```python
from build123d import *

# Parameters (mm, degrees)
ESQUISSE1_W             = 40
ESQUISSE1_H             = 40
BOSS_EXTRU_1_DEPTH      = 25
CHANFREIN1_SIZE         = 20
CHANFREIN1_SIZE2        = 11.547005384
ESQUISSE2_W             = 15
ESQUISSE2_H             = 15
ENL_V_MAT_EXTRU_1_DEPTH = 2


with BuildPart() as part:
    # Esquisse1 → Boss.-Extru.1 (new body)
    with BuildSketch(Plane(origin=(0, 0, 0), x_dir=(1, 0, 0), z_dir=(0, 1, 0))):
        Rectangle(ESQUISSE1_W, ESQUISSE1_H)
    extrude(amount=BOSS_EXTRU_1_DEPTH)

    # Chanfrein1
    chanfrein1_edges = [part.edges().sort_by_distance(p)[0] for p in [
        (20, 25, 0),
    ]]
    chanfrein1_side = [part.faces().sort_by_distance(p)[0] for p in [
        (20, 12.5, 0),
    ]]
    chamfer(chanfrein1_edges, length=CHANFREIN1_SIZE, length2=CHANFREIN1_SIZE2, reference=chanfrein1_side[0])

    # Esquisse2 → Enlèv. mat.-Extru.1 (cut)
    with BuildSketch(Plane(origin=(17.165063509, 9.910254038, 0), x_dir=(0, 0, -1), z_dir=(0.8660254037844397, 0.4999999999999983, 0))):
        with Locations((0, 5.877132403)):
            Rectangle(ESQUISSE2_W, ESQUISSE2_H)
    extrude(amount=-ENL_V_MAT_EXTRU_1_DEPTH, mode=Mode.SUBTRACT)


solid = part.part
```
Part model, mm, in its own coordinate system. A direction names the side the tool comes from. Round coordinates to 2 decimals unless told otherwise and drop trailing zeros. Loops run counter-clockwise (first coordinate to the right, second up) from the corner with the lowest first, then second, coordinate; pieces in that order, holes last. Notation, with made-up numbers: (18.25, 14.5) -> (66.25, 14.5) arc R6 cw to (66.25, 19.5) -> close; hole circle Ø2 at (3, 68). An arc over 180 degrees is marked (long way). Use CSV: the item, a comma, the result in double quotes. Start each with the question number.
1) Cut at B-B, the plane y = 17.5. Write the cut outline in (x, z), plus the area to 3 significant figures.
2) Cut at D-D, the plane z = -10. Write the cut outline in (x, y).
3) Pull direction Z, two halves, no side cores. Call faces 1 (the flat face through (13, 14, 7.5)), 2 (the flat face through (-20, 12, 0)), 3 (the flat face through (0, 12, 20)): +Z half, -Z half, draft (parallel to the pull), parting line (faces both ways), or undercut.
4) Drop a flat-ended pin along its axis: P1, Ø1, axis at y = 9, z = 14, coming from the +X side. Give the stop position or say it passes through.
5) Wall check: L1, parallel to Z at x = 13, y = 14; L2, parallel to X at y = 14.25, z = 7; L3, parallel to Y at x = 18, z = 14. Give the ranges that are in metal, low to high. Write a range as [from, to].
6) Cut at C-C, the plane x = 17. Write the cut outline in (y, z).
7) Cut at A-A, the plane z = -4.5. Write the cut outline in (x, y).
8) Which spindle directions (+Z, -Z, +X, -X, +Y, -Y) get a long thin tool onto all of the face, cutting with end or side? Do faces 4 (the flat face through (0, 12, -20)), 5 (the flat face through (17.1, 8, 0.1)), 6 (the flat face through (9.62, 21, 0.1)). Say none if no direction does.
Determined:
1,outline,"(-20, -20) -> (12.78, -20) -> (12.78, -7.5) -> (10.47, -7.5) -> (10.47, 7.5) -> (12.78, 7.5) -> (12.78, 20) -> (-20, 20) -> close"
1,area,"1,280 mm2"
2,outline,"(-20, 0) -> (20, 0) -> (20, 5) -> (8.45, 25) -> (-20, 25) -> close"
3,face 1,"undercut"
3,face 2,"draft"
3,face 3,"+Z half"
4,P1,"stops at x = 17.98"
5,L1,"z = [-20, -7.5], [7.5, 20]"
5,L2,"x = [-20, 12.35]"
5,L3,"y = [0, 8.46]"
6,outline,"(0, -20) -> (10.2, -20) -> (10.2, -7.5) -> (7.94, -7.5) -> (7.94, 7.5) -> (10.2, 7.5) -> (10.2, 20) -> (0, 20) -> close"
7,outline,"(-20, 0) -> (20, 0) -> (20, 5) -> (17.98, 8.5) -> (16.24, 7.5) -> (8.74, 20.5) -> (10.48, 21.5) -> (8.45, 25) -> (-20, 25) -> close"
8,face 4,"-Z, +X, -X, +Y, -Y"
8,face 5,"+Y"
8,face 6,"+X"
